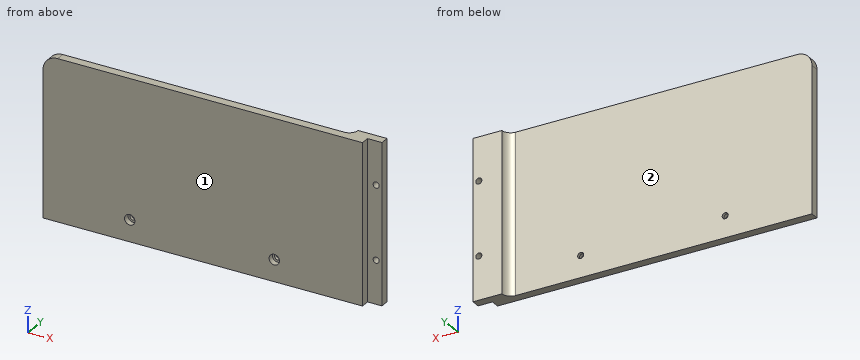
Autodesk Inventor part; units mm, degrees
ref_plane "YZ Plane" through (0, 0, 0) normal (1, 0, 0) x (0, 1, 0)
ref_plane "XZ Plane" through (0, 0, 0) normal (0, 1, 0) x (-1, 0, 0)
ref_plane "XY Plane" through (0, 0, 0) normal (0, 0, 1) x (1, 0, 0)
sketch "草图1" plane through (0, 0, 0) normal (0, 1, 0) x (-1, 0, 0)
  line L0 (110.5, 55.5) -> (-110.5, 55.5)
  line L1 (-110.5, 55.5) -> (-110.5, -55.5)
  line L2 (-110.5, -55.5) -> (110.5, -55.5)
  line L3 (110.5, -55.5) -> (110.5, 55.5)
  line L4 (0, 7.5575) -> (0, -11)
  line L5 (8.5019, 0) -> (-7, 0)
  point P0 (0, 0)
  dimension "d0" = 221
  dimension "d1" = 111
extrude "拉伸1" add sketch "草图1" along normal blind 6
fillet "圆角1" radius 10.1 1 edges at (-110.5, 3, 55.5)
sketch "草图2" plane through (0, 6, 0) normal (0, 1, 0) x (1, 0, 0)
  line L0 (110.5, 55.5) -> (-110.5, 55.5)
  line L1 (100.5, 55.5) -> (120.5, 55.5)
  line L2 (120.5, 55.5) -> (120.5, -55.5)
  line L3 (120.5, -55.5) -> (100.5, -55.5)
  line L4 (100.5, -55.5) -> (100.5, 55.5)
  line L5 (110.5, -55.5) -> (110.5, 55.5)
  line L6 (-100.4, -55.5) -> (110.5, -55.5)
  circle A0 centre (116.5, 25.5) radius 2.1
  circle A1 centre (116.5, -25.5) radius 2.1
  point P0 (0, 0)
  dimension "d5" = 20
  dimension "d6" = 10
  dimension "d7" = 4.2
  dimension "d8" = 4.2
  dimension "d9" = 4
  dimension "d10" = 4
  dimension "d11" = 30
  dimension "d12" = 30
extrude "拉伸2" add sketch "草图2" along normal blind 6
fillet "圆角2" radius 6 1 edges at (100.5, 6, 0)
sketch "草图3" plane through (0, 0, 0) normal (0, -1, 0) x (1, 0, 0)
  circle A0 centre (-50.5, -40.5) radius 2.1
  circle A1 centre (49.5, -40.5) radius 2.1
  line L0 (110.5, -55.5) -> (-110.5, -55.5)
  line L1 (-110.5, -55.5) -> (-110.5, 45.4)
  point P0 (0, 0)
  dimension "d16" = 4.2
  dimension "d17" = 4.2
  dimension "d18" = 15
  dimension "d19" = 15
  dimension "d20" = 60
  dimension "d21" = 100
extrude "拉伸3" cut sketch "草图3" against normal blind 10
sketch "草图4" plane through (0, 0, 0) normal (0, -1, 0) x (1, 0, 0)
  circle A0 centre (-50.5, -40.5) radius 2.1
  circle A1 centre (-50.5, -40.5) radius 3.6
  circle A2 centre (49.5, -40.5) radius 2.1
  circle A3 centre (49.5, -40.5) radius 3.6
  point P0 (0, 0)
  dimension "d24" = 7.2
  dimension "d25" = 7.2
extrude "拉伸4" cut sketch "草图4" against normal blind 4 contours A0 | A1 | A2 | A3
properties part number "底板_A"
Part model, mm, in its own coordinate system. Face numbers are marked on the shaded views. A direction names the side the tool comes from. Round coordinates to 2 decimals unless told otherwise and drop trailing zeros. Loops run counter-clockwise (first coordinate to the right, second up) from the corner with the lowest first, then second, coordinate; pieces in that order, holes last.
Item 1: Drop flat-ended pins along their axis: P1, Ø2, axis at x = 7, z = -31, coming from the +Y side; P2, Ø5.5, axis at x = -50.5, z = -40.5, coming from the -Y side; P3, Ø8, axis at x = 115, z = -12, coming from the -Y side; P4, Ø1, axis at x = -69.5, y = 7, coming from the -Z side. Give the stop position or say it passes through.
Item 2: Cut at B-B, the plane x = 49.5. Give the cut face in (y, z).
Item 3: 3-axis set-ups, long thin cutter, end or side, ignore diameter. For the marked faces 1 and 2: which of +Z, -Z, +X, -X, +Y, -Y reach the whole face in a straight line?
Item 4: Drill centre lines: line 1 (Z direction, x = 116.5, y = 7.65); line 2 (Z direction, x = -50.5, y = 5.4); line 3 (X direction, y = 5, z = 38.5). Where is each one in solid material? Low to high.
Item 5: Cut at C-C, the plane z = -40.5. State how many separate pieces and enclosed holes the cut face has, then the cut area to 3 significant figures.
Item 6: Cut at D-D, the plane y = 2. Give the cut face in (x, z), then the cut area to 3 significant figures.
A:
1. P1: stops at y = 6
1. P2: stops at y = 4
1. P3: stops at y = 6
1. P4: passes through
2. outline: (0, -55.5) - (6, -55.5) - (6, -42.6) - (4, -42.6) - (4, -44.1) - (0, -44.1) - close; (0, -36.9) - (4, -36.9) - (4, -38.4) - (6, -38.4) - (6, 55.5) - (0, 55.5) - close
3. face 1: +Z, -Z, +X, -X, -Y
3. face 2: +Z, -Z, -X, +Y
4. line 1: z = -55.5 to -27.6, -23.4 to 23.4, 27.6 to 55.5
4. line 2: z = -55.5 to -42.6, -38.4 to 55.5
4. line 3: x = -110.5 to 110.5
5. separate pieces: 3
5. enclosed holes: 0
5. area: 1,380 mm2
6. outline: (-110.5, -55.5) - (110.5, -55.5) - (110.5, 55.5) - (-100.4, 55.5) arc R10.1 ccw to (-110.5, 45.4) - close; hole circle Ø7.2 at (-50.5, -40.5); hole circle Ø7.2 at (49.5, -40.5)
6. area: 24,400 mm2
